The listing builds one solid part. Answer for the finished solid, in the listing's coordinates (mm). Give positions to 0.01 mm unless a question says otherwise; leave off trailing zeros. Write each loop counter-clockwise with the first axis right and the second up, starting at its lowest first coordinate (ties: lowest second). Pieces come first, ordered by that corner, then holes. Notation, with made-up numbers: (21.5, 9) - (28.5, 9) arc R18 ccw to (28.5, 37) - close; hole circle Ø7 at (30.25, -9). An arc over 180 degrees is marked (long way). Return JSON: item names as keys, results as strings.
from build123d import *

# Parameters (mm, degrees)
F1_R     = 25.4
F1_R_2   = 22.225
F2_DEPTH = 1625.6
F4_DEPTH = 50


with BuildPart() as f2:
    # F1 (on Top) → F2 (new body)
    with BuildSketch(Plane.XY):
        Circle(F1_R)
        Circle(F1_R_2, mode=Mode.SUBTRACT)
    extrude(amount=F2_DEPTH)

    # F3 (on Front) → F4 (cut)
    with BuildSketch(Plane.XZ):
        with BuildLine():
            ThreePointArc((12.3654246976, 328.0673227027), (1.1899269468, 340.763681787), (-13.0896388975, 331.698182172))
            Line((-13.0896388975, 331.698182172), (-12.3654246976, 281.5326772973))
            ThreePointArc((-12.3654246976, 281.5326772973), (-1.7614192029, 264.8297264279), (13.0896388975, 277.901817828))
            Line((13.0896388975, 277.901817828), (12.3654246976, 328.0673227027))
        make_face()
        with BuildLine():
            ThreePointArc((-17.8609726221, 1293.9123234562), (-3.4922049716, 1284.9888824058), (7.5568313695, 1297.7954463442))
            Line((7.5568313695, 1297.7954463442), (7.7835105534, 1347.9656664163))
            ThreePointArc((7.7835105534, 1347.9656664163), (-7.1964552661, 1360.8898346418), (-17.6342934381, 1344.0825435284))
            Line((-17.6342934381, 1344.0825435284), (-17.8609726221, 1293.9123234562))
        make_face()
    extrude(amount=F4_DEPTH, mode=Mode.SUBTRACT)


solid = f2.part
Item 1: A cutting plane is placed at B-B on z = 191.5. Determine the outline of the cut face in (x, y) (3 decimals).
Answer below:
{"outline": "circle Ø50.8 at (0, 0); hole circle Ø44.45 at (0, 0)"}
Item 2: The mould has two halves that part along Y. Classify faces 1 (the face through (-0.1, -22.5, 0)), 2 (the face through (11.95, 18.74, 801.42)), 3 (the face through (-3.307, 25.184, 801.421)): +Y half, -Y half, draft (parallel to the pull), parting line (faces both ways), or undercut.
Answer below:
{"face 1": "draft", "face 2": "undercut", "face 3": "parting line"}
Item 3: Consider L1, parallel to Y at x = 0, z = 861 (3 decimals); L2, parallel to X at y = -1, z = 1211; L3, parallel to Y at x = -7, z = 496. Determine where each line is inside the solid, lowest interval first.
Answer below:
{"L1": "y = -25.4 to -22.225, 22.225 to 25.4", "L2": "x = -25.38 to -22.2, 22.2 to 25.38", "L3": "y = -24.42 to -21.09, 21.09 to 24.42"}
Item 4: Flat-ended cylindrical pins translate along their axes: P1, Ø1.5, axis at x = -19.5, y = -13.5, coming from the -Z side; P2, Ø8, axis at x = 2.5, y = 16.5, coming from the +Z side; P3, Ø5, axis at y = 15.5, z = 1095, coming from the -X side; P4, Ø15.5, axis at x = -5.23, z = 1348.02, coming from the +Y side. Find the tip coordinate at first contact, or state that the pin passes through.
Answer below:
{"P1": "stops at z = 0", "P2": "passes through", "P3": "stops at x = -21.82", "P4": "stops at y = 25.4"}
Item 5: A cutting plane is placed at A-A on y = 0. Determine the outline of the cut face in (x, z) (3 decimals).
Answer below:
{"outline": "(-25.4, 0) - (-22.225, 0) - (-22.225, 1625.6) - (-25.4, 1625.6) - close; (22.225, 0) - (25.4, 0) - (25.4, 1625.6) - (22.225, 1625.6) - close"}
